from build123d import *

# Parameters (mm, degrees)
SKETCH1_R          = 5.55625
EXTRUDE1_DEPTH     = 25.4
SKETCH2_R          = 3.175
EXTRUDE2_DEPTH     = 9.525
CHAMFER1_SIZE      = 1.5875
CUT_EXTRUDE1_DEPTH = 1.5875


with BuildPart() as part:
    # Sketch1 → Extrude1 (new body)
    with BuildSketch(Plane.XY):
        Circle(SKETCH1_R)
    extrude(amount=EXTRUDE1_DEPTH)

    # Sketch2 → Extrude2 (add)
    with BuildSketch(Plane.XY.offset(25.4)):
        Circle(SKETCH2_R)
    extrude(amount=EXTRUDE2_DEPTH)

    # Chamfer1
    chamfer1_edges = [part.edges().sort_by_distance(p)[0] for p in [
        (-5.55625, 0, 0),
        (-5.55625, 0, 25.4),
        (-3.175, 0, 34.925),
    ]]
    chamfer(chamfer1_edges, length=CHAMFER1_SIZE)

    # Sketch3 → Cut-Extrude1 (cut, symmetric)
    with BuildSketch(Plane(origin=(0, 0, 0), x_dir=(1, 0, 0), z_dir=(0, 1, 0))):
        with BuildLine():
            Line((3.77825, -9.623700346), (3.77825, -25.4))
            Line((3.77825, -25.4), (5.55625, -25.4))
            Line((5.55625, -25.4), (5.55625, -1.5875))
            ThreePointArc((5.55625, -1.5875), (4.228060485, -5.508430002), (3.77825, -9.623700346))
        make_face()
    extrude(amount=CUT_EXTRUDE1_DEPTH, both=True, mode=Mode.SUBTRACT)


solid = part.part
Geometry: final body of the model. Coordinates: model frame, mm. A direction names the side the tool comes from. Give positions to 0.01 mm unless a question says otherwise; leave off trailing zeros. Loops run counter-clockwise (first coordinate to the right, second up) from the corner with the lowest first, then second, coordinate; pieces in that order, holes last. Notation, with made-up numbers: (10, 56) - (30, 56) arc R28 cw to (30, 78) - close; hole circle Ø2 at (41, 49.5). An arc over 180 degrees is marked (long way). One line per question, with ' | ' between items. Start each with the question number.
(1) Contact query for flat-ended pins moving along their axis: pin 1 (2 mm diameter, centred on x = 3.5, z = 7.5, fed in from +Y); pin 2 (1.6 mm diameter, centred on y = -0.5, z = 14, fed in from +X); pin 3 (1.5 mm diameter, centred on x = 1.5, y = -2.5, fed in from +Z); pin 4 (5 mm diameter, centred on x = 2.5, y = 2.5, fed in from -Z). Output: stop coordinate, or through.
(2) Section query A-A on x = 0. Return loops of the section in (y, z) (1 decimal), then the cut area to 3 significant figures.
(3) Reachability of faces 1 (the flat face through (3.778, 0, 17)), 2 (the flat face through (0, 0, 34.925)), 3 (the flat face through (-2, 3, 25.4)) from +Z, -Z, +X, -X, +Y, -Y: full face, straight path, thin tool, end or side. Return the list, or none.
(4) Pull-direction query (Y, two-part tool) for faces 4 (the cylindrical face through (4.24, 0.02, 5.45)), 5 (the cylindrical face through (-0.69, -3.1, 29.31)), 6 (the flat face through (0, 0, 0)); classes: released by +Y, released by -Y, zero draft, split by the parting line, or undercut.
(5) Section query B-B on z = 33. Return loops of the section in (x, y) (3 decimals).
(6) Ray query, line 1 (Z direction, x = -2.5, y = 2.75); line 2 (Y direction, x = 4.25, z = 15); line 3 (X direction, y = 3.25, z = 18.5). Return the intervals inside material, ascending. Write a range as from..to.
(7) Section query C-C on z = 23.5. Return loops of the section in (x, y), then the cut area to 3 significant figures.
The answers:
1) pin 1: y = 4.96 | pin 2: x = 3.78 | pin 3: z = 34.35 | pin 4: z = 0
2) outline: (-5.6, 1.6) - (-4, 0) - (4, 0) - (5.6, 1.6) - (5.6, 23.8) - (4, 25.4) - (3.2, 25.4) - (3.2, 33.3) - (1.6, 34.9) - (-1.6, 34.9) - (-3.2, 33.3) - (-3.2, 25.4) - (-4, 25.4) - (-5.6, 23.8) - close | area: 335 mm2
3) face 1: +Z, +X | face 2: +Z, +X, -X, +Y, -Y | face 3: +Z
4) face 4: undercut | face 5: split by the parting line | face 6: zero draft
5) outline: circle Ø6.35 at (0, 0)
6) line 1: 0..25.4 | line 2: -3.58..-1.59, 1.59..3.58 | line 3: -4.51..4.51
7) outline: (3.78, -1.59) - (3.78, 1.59) - (5.32, 1.59) arc R5.56 ccw (long way) to (5.32, -1.59) - close | area: 91.6 mm2
